```python
from build123d import *

# Parameters (mm, degrees)
SKETCH1_R            = 9.5
SKETCH1_R_2          = 3
BOSS_EXTRUDE1_DEPTH  = 3
SKETCH7_R            = 8.5
SKETCH7_R_2          = 3
BOSS_EXTRUDE5_DEPTH  = 8.4
SKETCH8_R            = 9.5
SKETCH8_R_2          = 8.5
BOSS_EXTRUDE6_DEPTH  = 3.5
CHAMFER1_SIZE        = 1.5
SKETCH12_R           = 3
SKETCH12_R_2         = 1
CUT_EXTRUDE4_DEPTH   = 18.978668035
M3_CLEARANCE_HOLE1_D = 3.4
CHAMFER2_SIZE        = 0.3


with BuildPart() as part:
    # Sketch1 → Boss-Extrude1 (new body)
    with BuildSketch(Plane(origin=(0, 0, 0), x_dir=(1, 0, 0), z_dir=(0, 1, 0))):
        with Locations(Location((-0.65, 0, 0), (0, 0, 270))):
            Circle(SKETCH1_R)
        with Locations(Location((0, 0, 0), (0, 0, 270))):
            Circle(SKETCH1_R_2, mode=Mode.SUBTRACT)
    extrude(amount=BOSS_EXTRUDE1_DEPTH)

    # Sketch7 → Boss-Extrude5 (add)
    with BuildSketch(Plane(origin=(0, 3, 0), x_dir=(1, 0, 0), z_dir=(0, 1, 0))):
        with Locations(Location((0.65, 0, 0), (0, 0, 42.437907805))):
            Circle(SKETCH7_R)
        with Locations(Location((0, 0, 0), (0, 0, 270))):
            Circle(SKETCH7_R_2, mode=Mode.SUBTRACT)
    extrude(amount=BOSS_EXTRUDE5_DEPTH)

    # Sketch8 → Boss-Extrude6 (add)
    with BuildSketch(Plane(origin=(0, 3, 0), x_dir=(1, 0, 0), z_dir=(0, 1, 0))):
        with Locations(Location((0.65, 0, 0), (0, 0, 93.923302734))):
            Circle(SKETCH8_R)
        with Locations(Location((0.65, 0, 0), (0, 0, 270))):
            Circle(SKETCH8_R_2, mode=Mode.SUBTRACT)
    extrude(amount=BOSS_EXTRUDE6_DEPTH)

    # Chamfer1
    # the kernel refuses this chamfer: 1.5 mm, written as the material it adds along each edge
    with BuildSketch(Plane(origin=(-0.65, 3, 0), x_dir=(-0.3317687677714116, 0, -0.9433607394477679), z_dir=(-0.9433607394477679, 0, 0.3317687677714116))) as chamfer1_piece_1_section:
        Polygon((9.5, CHAMFER1_SIZE), (9.5 + CHAMFER1_SIZE, 0), (9.5, 0), align=None)
    chamfer1_piece_1 = revolve(axis=Axis((-0.65, 3, 0), (0, -1, 0)), revolution_arc=218.752335407, mode=Mode.PRIVATE)
    chamfer1_piece_1 = chamfer1_piece_1 & Plane(origin=(0.65, 2.170447869, 0), x_dir=(-0.06842105263614455, 0, -0.9976565338613094), z_dir=(0, -1, 0)) * Cylinder(9.5, 44, mode=Mode.PRIVATE)
    add(chamfer1_piece_1)

    # Sketch12 → Cut-Extrude4 (cut, through all)
    with BuildSketch(Plane(origin=(0, 11.4, 0), x_dir=(1, 0, 0), z_dir=(0, 1, 0))):
        with Locations(Location((0, 0, 0), (0, 0, 270))):
            Circle(SKETCH12_R)
        with Locations(Location((-5, 0, 0), (0, 0, 270))):
            Circle(SKETCH12_R_2)
    extrude(amount=-CUT_EXTRUDE4_DEPTH, mode=Mode.SUBTRACT)

    # M3 Clearance Hole1 (through all)
    with Locations(Plane(origin=(0, 11.4, 0), x_dir=(1, 0, 0), z_dir=(0, 1, 0))):
        with Locations((0, 6), (0, -6)):
            Hole(M3_CLEARANCE_HOLE1_D / 2)

    # Chamfer2
    chamfer2_edges = [part.edges().sort_by_distance(p)[0] for p in [
        (0, 11.4, -3),
        (-5, 0, -1),
        (-5, 11.4, -1),
        (0, 0, -3),
        (1.7, 11.4, 6),
        (1.7, 0, 6),
        (1.7, 11.4, -6),
        (1.7, 0, -6),
    ]]
    chamfer(chamfer2_edges, length=CHAMFER2_SIZE)


solid = part.part
```
Design review of the part built by this model. Coordinates are the model's own, in mm. A direction names the side the tool comes from. Round coordinates to 2 decimals unless told otherwise and drop trailing zeros. Write each loop counter-clockwise with the first axis right and the second up, starting at its lowest first coordinate (ties: lowest second). Pieces come first, ordered by that corner, then holes.
Item 1: We need section A-A on z = 0. Write out the cut boundary in (x, y), and give its area (3 significant figures).
Item 2: We need section D-D on x = -0.65. State how many separate pieces and enclosed holes the cut face has, and give its area (3 significant figures).
Item 3: For probe 1 along X at (y, z) = (4, 0); probe 2 along X at (y, z) = (8.5, 0); probe 3 along Z at (x, y) = (1.5, 9.25), list the stretches that pass through material, from the lowest coordinate up.
Item 4: We need section B-B on x = -5. Write out the cut boundary in (y, z), and give its area (3 significant figures).
Item 5: The part is to be moulded in two halves that separate along X. For faces 4 (the cylindrical face through (0.9, 5.62, 2.86)), 5 (the cylindrical face through (0.37, 5.62, 7.66)), 6 (the flat face through (6, 6.5, 7)), 7 (the conical face through (9.074, 1.726, -0.205)), say which applies: +X half, -X half, draft (parallel to the pull), parting line (faces both ways), or undercut.
Item 6: Clearance check with flat-ended pins moving along their axes: pin 1 Ø1 at (y, z) = (8, 4.5) entering from +X; pin 2 Ø1.5 at (x, y) = (-4, 8) entering from -Z; pin 3 Ø2.5 at (x, z) = (-5, 0) entering from -Y. State where each tip first meets the part, or that it passes through.
Item 7: For faces 1 (the cylindrical face through (8.64, 8.92, -2.9)), 2 (the cylindrical face through (-9.924, 1.146, -2.059)), 3 (the flat face through (-9, 3, 0)), list the 3-axis set-ups (+Z, -Z, +X, -X, +Y, -Y) from which the entire face can be reached by the end or side of a thin tool; tool diameter is ignored.
Item 8: We need section C-C on y = 8.75. Write out the cut boundary in (x, z), and give its area (3 significant figures).
Returned:
1. outline: (-10.15, 0) - (-6.3, 0) - (-6, 0.3) - (-6, 11.1) - (-6.3, 11.4) - (-7.85, 11.4) - (-7.85, 6.5) - (-8.85, 6.5) - (-8.85, 3) - (-10.15, 3) - close; (-4, 0.3) - (-3.7, 0) - (-3.3, 0) - (-3, 0.3) - (-3, 11.1) - (-3.3, 11.4) - (-3.7, 11.4) - (-4, 11.1) - close; (3, 0.3) - (3.3, 0) - (8.85, 0) - (8.85, 1.5) - (10.15, 2.8) - (10.15, 6.5) - (9.15, 6.5) - (9.15, 11.4) - (3.3, 11.4) - (3, 11.1) - close
1. area: 116 mm2
2. separate pieces: 4
2. enclosed holes: 0
2. area: 66.2 mm2
3. probe 1: x = -8.85 to -6, -4 to -3, 3 to 10.15
3. probe 2: x = -7.85 to -6, -4 to -3, 3 to 9.15
3. probe 3: z = -8.46 to -6.8, -5.2 to -2.6, 2.6 to 5.2, 6.8 to 8.46
4. outline: (0, -8.45) - (3, -8.45) - (3, -7.64) - (6.5, -7.64) - (6.5, -6.35) - (11.4, -6.35) - (11.4, -1.3) - (11.1, -1) - (0.3, -1) - (0, -1.3) - close; (0, 1.3) - (0.3, 1) - (11.1, 1) - (11.4, 1.3) - (11.4, 6.35) - (6.5, 6.35) - (6.5, 7.64) - (3, 7.64) - (3, 8.45) - (0, 8.45) - close
4. area: 143 mm2
5. face 4: undercut
5. face 5: undercut
5. face 6: draft
5. face 7: +X half
6. pin 1: stops at x = 8.15
6. pin 2: stops at z = -7.55
6. pin 3: stops at y = 0.05
7. face 1: +Y
7. face 2: -Y
7. face 3: -X, +Y
8. outline: circle Ø17 at (0.65, 0); hole circle Ø2 at (-5, 0); hole circle Ø6 at (0, 0); hole circle Ø3.4 at (0, -6); hole circle Ø3.4 at (0, 6)
8. area: 177 mm2
